Model file for the job. Use its own axes, mm. A direction names the side the tool comes from. Round coordinates to 2 decimals unless told otherwise and drop trailing zeros. Write each loop counter-clockwise with the first axis right and the second up, starting at its lowest first coordinate (ties: lowest second). Pieces come first, ordered by that corner, then holes.
```python
from build123d import *

# Parameters (mm, degrees)
F0_R      = 10.95
F1_DEPTH  = 2.4
F2_R      = 4
F3_DEPTH  = 4.2
F4_R      = 1
F5_R      = 5.2
F5_R_2    = 4
F6_DEPTH  = 1
F7_R      = 1
F8_R      = 8.5
F9_DEPTH  = 2
F11_SIZE  = 0.4
F12_R     = 3
F13_R     = 2.4
F14_DEPTH = 2.5


# Not quite as in the source:
# - a fillet or chamfer that OpenCascade refuses, or shapes differently, is made with other operations: its cross-section is extruded or revolved along the edge and cut away or added


with BuildPart() as f1:
    # F0 (on Top) → F1 (new body)
    with BuildSketch(Plane.XY):
        Circle(F0_R)
    extrude(amount=F1_DEPTH)

    # F2 (on face) → F3 (join)
    with BuildSketch(Plane.XY.offset(2.4)):
        Circle(F2_R)
    extrude(amount=F3_DEPTH)

    # F4
    f4_edges = [f1.edges().sort_by_distance(p)[0] for p in [
        (-10.95, 0, 2.4),
    ]]
    fillet(f4_edges, radius=F4_R)

    # F5 (on face) → F6 (join)
    with BuildSketch(Plane.XY.offset(2.4)):
        Circle(F5_R)
        Circle(F5_R_2, mode=Mode.SUBTRACT)
    extrude(amount=F6_DEPTH)

    # F7
    f7_edges = [f1.edges().sort_by_distance(p)[0] for p in [
        (-10.95, 0, 0),
    ]]
    fillet(f7_edges, radius=F7_R)

    # F8 (on face) → F9 (cut)
    with BuildSketch(Plane(origin=(0, 0, 0), x_dir=(1, 0, 0), z_dir=(0, 0, -1))):
        Circle(F8_R)
    extrude(amount=-F9_DEPTH, mode=Mode.SUBTRACT)

    # F10: fillet of radius 9 on 1 edges, made by hand

    # F10_s1 → F10_t2 (revolve)
    with BuildSketch(Plane.XZ):
        with BuildLine():
            ThreePointArc((8.5, 0), (5.8431457505, 1.4852813742), (2.8431457505, 2))
            Line((2.8431457505, 2), (8.5, 2))
            Line((8.5, 2), (8.5, 0))
        make_face()
    revolve(axis=Axis((0, 0, 2), (0, 0, -1)))

    # F11
    f11_edges = [f1.edges().sort_by_distance(p)[0] for p in [
        (-4, 0, 6.6),
    ]]
    chamfer(f11_edges, length=F11_SIZE)

    # F12
    f12_edges = [f1.edges().sort_by_distance(p)[0] for p in [
        (-8.5, 0, 0),
    ]]
    fillet(f12_edges, radius=F12_R)

    # F13 (on face) → F14 (cut)
    with BuildSketch(Plane.XY.offset(6.6)):
        Circle(F13_R)
    extrude(amount=-F14_DEPTH, mode=Mode.SUBTRACT)


solid = f1.part
```
1) Cut at A-A on z = 5.75. List the corners of the cut face in (x, y), and give its area (3 significant figures).
2) Which spindle directions (+Z, -Z, +X, -X, +Y, -Y) get a long thin tool onto all of the face, cutting with end or side? Do faces 4 (the face through (-8.69, -6.66, 1.2)), 5 (the face through (1.29, 2.024, 5.368)). Say none if no direction does.
3) Flat gauge pins, fed straight in: pin 1 Ø3 at (x, z) = (-7, 3.5) entering from -Y; pin 2 Ø4.5 at (x, y) = (0, 0) entering from +Z; pin 3 Ø6.5 at (x, y) = (0.5, 0.5) entering from -Z. Where does each tip first touch, or does it go through?
4) Pull direction Y, two halves, no side cores. Call faces 1 (the face through (-0.677, 5.156, 2.893)), 2 (the face through (0, 0, 2)), 3 (the face through (3, -3, 3.4)): released by +Y, released by -Y, zero draft, split by the parting line, or undercut.
5) Wall check: probe 1 along Y at (x, z) = (0, 6.1); probe 2 along Z at (x, y) = (-9, -4); probe 3 along Z at (x, y) = (2, -0.75). Give the ranges that are in metal, low to high.
Result sheet:
1. outline: circle Ø8 at (0, 0); hole circle Ø4.8 at (0, 0)
1. area: 32.2 mm2
2. face 4: +Z, -Z
2. face 5: +Z
3. pin 1: stops at y = -8.51
3. pin 2: stops at z = 4.1
3. pin 3: stops at z = 1.93
4. face 1: split by the parting line
4. face 2: undercut
4. face 3: zero draft
5. probe 1: y = -4 to -2.4, 2.4 to 4
5. probe 2: z = 0 to 2.4
5. probe 3: z = 2 to 4.1
